from build123d import *

# Parameters (mm, degrees)
PAD_DEPTH       = 105
PAD_DEPTH_BACK  = 105
SKETCH001_R     = 1.65
SKETCH001_W     = 38.25
SKETCH001_H     = 51.5
POCKET_DEPTH    = 101.705966
SKETCH003_R     = 1.65
POCKET001_DEPTH = 5
SKETCH004_W     = 2
SKETCH004_H     = 210
PAD001_DEPTH    = 5
FILLET_R        = 1
SKETCH005_R     = 10
POCKET002_DEPTH = 5


with BuildPart() as part:
    # Sketch → Pad (new body, two sides)
    with BuildSketch(Plane.YZ) as pad_sk:
        with BuildLine():
            Line((12.736792, 82.5), (57.500792, 82.5))
            Line((57.500792, 82.5), (57.500792, 80))
            Line((57.500792, 80), (12.736792, 80))
            ThreePointArc((12.736792, 80), (-1.613837, 77.145482), (-13.779712, 69.016504))
            Line((-13.779712, 69.016504), (-43.478197, 39.318019))
            ThreePointArc((-43.478197, 39.318019), (-52.006167, 26.55501), (-55.000792, 11.500014))
            Line((-55.000792, 11.500014), (-55.000792, 0))
            Line((-55.000792, 0), (-57.500792, 0))
            Line((-57.500792, 11.500014), (-57.500792, 0))
            ThreePointArc((-45.245964, 41.085786), (-54.315866, 27.511719), (-57.500792, 11.500014))
            Line((-15.547479, 70.784271), (-45.245964, 41.085786))
            ThreePointArc((12.736792, 82.5), (-2.570545, 79.455181), (-15.547479, 70.784271))
        make_face()
    extrude(amount=PAD_DEPTH)
    extrude(pad_sk.sketch, amount=-PAD_DEPTH_BACK)

    # Sketch001 (on Face12 of Pad) → Pocket (cut, through all)
    with BuildSketch(Plane(origin=(0, -43.165875, 43.165875), x_dir=(0, -0.707107, -0.707107), z_dir=(0, -0.707107, 0.707107))):
        with Locations((-34.55831, 28.7)):
            Circle(SKETCH001_R)
        with Locations((-1.55831, 28.7)):
            Circle(SKETCH001_R)
        with Locations((-34.55831, -28.7)):
            Circle(SKETCH001_R)
        with Locations((-1.55831, -28.7)):
            Circle(SKETCH001_R)
        with Locations((-18.05831, 0)):
            Rectangle(SKETCH001_W, SKETCH001_H)
    extrude(amount=-POCKET_DEPTH, mode=Mode.SUBTRACT)

    # Sketch003 (on Face2 of Pocket) → Pocket001 (cut)
    with BuildSketch(Plane(origin=(0, 0, 82.5), x_dir=(0, -1, 0), z_dir=(0, 0, 1))):
        with Locations((-47.500792, 15)):
            Circle(SKETCH003_R)
        with Locations((-47.500792, 45)):
            Circle(SKETCH003_R)
        with Locations((-47.500792, -15)):
            Circle(SKETCH003_R)
        with Locations((-47.500792, -45)):
            Circle(SKETCH003_R)
        with Locations((-47.500792, 60)):
            Circle(SKETCH003_R)
        with Locations((-47.500792, -60)):
            Circle(SKETCH003_R)
    extrude(amount=-POCKET001_DEPTH, mode=Mode.SUBTRACT)

    # Sketch004 (on Face26 of Pocket001) → Pad001 (join)
    with BuildSketch(Plane.ZX.offset(-55.000792)):
        with Locations((1, 0)):
            Rectangle(SKETCH004_W, SKETCH004_H)
    extrude(amount=PAD001_DEPTH)

    # Fillet
    fillet_edges = [part.edges().sort_by_distance(p)[0] for p in [
        (0, -55.000792, 2),
    ]]
    fillet(fillet_edges, radius=FILLET_R)

    # Sketch005 (on Face15 of Fillet) → Pocket002 (cut)
    with BuildSketch(Plane(origin=(0, 0, 82.5), x_dir=(0, -1, 0), z_dir=(0, 0, 1))):
        with Locations((-27.500792, 0)):
            Circle(SKETCH005_R)
    extrude(amount=-POCKET002_DEPTH, mode=Mode.SUBTRACT)


solid = part.part
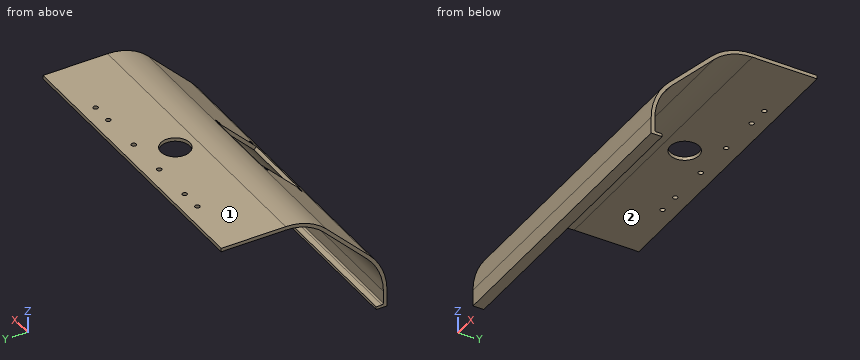
The listing builds one solid part. Answer for the finished solid, in the listing's coordinates (mm). Face numbers are marked on the shaded views. A direction names the side the tool comes from. Coordinates: 2 decimals unless noted, no trailing zeros. Write each loop counter-clockwise with the first axis right and the second up, starting at its lowest first coordinate (ties: lowest second). Pieces come first, ordered by that corner, then holes. Notation, with made-up numbers: (77, 34) - (121, 34) arc R20 cw to (121, 62) - close; hole circle Ø1 at (-11.75, -28). An arc over 180 degrees is marked (long way). Answer as CSV lines item,"result".
1. Find section D-D (z = 77). Give the vertices of the cut face in (x, y).
Computed values:
outline,"(-105, -7.51) - (105, -7.51) - (105, -1.96) - (-105, -1.96) - close"
2. Find section A-A (x = 0). Give the vertices of the cut face in (y, z), plus the area to 3 significant figures.
Computed values:
outline,"(-57.5, 0) - (-50, 0) - (-50, 2) - (-54, 2) arc R1 cw to (-55, 3) - (-55, 11.5) arc R39.34 cw to (-43.48, 39.32) - (-42.15, 40.64) - (-43.92, 42.41) - (-45.25, 41.09) arc R41.84 ccw to (-57.5, 11.5) - close; (-16.87, 69.46) - (-15.11, 67.69) - (-13.78, 69.02) arc R37.5 cw to (12.74, 80) - (17.5, 80) - (17.5, 82.5) - (12.74, 82.5) arc R40 ccw to (-15.55, 70.78) - close; (37.5, 80) - (57.5, 80) - (57.5, 82.5) - (37.5, 82.5) - close"
area,"266 mm²"
3. A tool of negligible diameter and unlimited length cuts with its end or side. For the marked faces 1 and 2, from which of +Z, -Z, +X, -X, +Y, -Y can it reach the whole face along a straight path? Write none if from no direction.
Computed values:
face 1,"+Z, +X, -X, +Y, -Y"
face 2,"-Z, +X, -X, +Y"
4. Straight lines are drawn through the part: line 1 (Y direction, x = -30, z = 22); line 2 (Z direction, x = -43, y = -30); line 3 (Z direction, x = 66, y = -43.5). For each, find the intervals that lie inside material, in ascending order. Write a range as [from, to].
Computed values:
line 1,"y = [-56.16, -53.57]"
line 2,"z = [52.8, 56.33]"
line 3,"z = [39.3, 42.83]"
5. Find section B-B (y = 32.5). Give the vertices of the cut face in (x, z).
Computed values:
outline,"(-105, 80) - (-8.66, 80) - (-8.66, 82.5) - (-105, 82.5) - close; (8.66, 80) - (105, 80) - (105, 82.5) - (8.66, 82.5) - close"
6. Find section C-C (x = -23). Give the vertices of the cut face in (y, z).
Computed values:
outline,"(-57.5, 0) - (-50, 0) - (-50, 2) - (-54, 2) arc R1 cw to (-55, 3) - (-55, 11.5) arc R39.34 cw to (-43.48, 39.32) - (-42.15, 40.64) - (-43.92, 42.41) - (-45.25, 41.09) arc R41.84 ccw to (-57.5, 11.5) - close; (-16.87, 69.46) - (-15.11, 67.69) - (-13.78, 69.02) arc R37.5 cw to (12.74, 80) - (57.5, 80) - (57.5, 82.5) - (12.74, 82.5) arc R40 ccw to (-15.55, 70.78) - close"
7. Given P1, Ø2.5, axis at x = -45, y = 47.5, coming from the +Z side; P2, Ø8, axis at x = 36.5, z = 24, coming from the -Y side; P3, Ø4, axis at x = 15, y = 47.5, coming from the +Z side; P4, Ø4.5, axis at x = 45, y = -52.5, coming from the +Z side, each flat-ended and moving along its own axis, determine where each tip first touches the part or whether it passes through.
Computed values:
P1,"passes through"
P2,"stops at y = -56.63"
P3,"stops at z = 82.5"
P4,"stops at z = 35.04"
